Input: part model. Units: mm. Frame: model coordinates. A direction names the side the tool comes from. Give positions to 0.01 mm unless a question says otherwise; leave off trailing zeros. Loops run counter-clockwise (first coordinate to the right, second up) from the corner with the lowest first, then second, coordinate; pieces in that order, holes last. Notation, with made-up numbers: M 49.5,71 L 108.5,71 A21 ccw 108.5,104 Z; hole C -30.75,71.5 d2. An arc over 180 degrees is marked long. One line per item, written item: value. Start each with the question number.
(1) Access query for faces 4 (the flat face through (0, -27.5, 1)), 5 (the flat face through (32.5, 0, -12)), 6 (the flat face through (-47, 0, -20)), 7 (the cylindrical face through (-2.38, -10.74, 2.54)), 8 (the flat face through (37.5, 0, -7)). Directions: +Z, -Z, +X, -X, +Y, -Y. A direction counts if a zero-diameter tool reaches every point of the face in a straight line with its end or side. Return the directions, or none.
(2) Section B-B on z = -12.25. Output: boundary loops of the cut face in (x, y).
(3) Pull-direction query (X, two-part tool) for faces 1 (the flat face through (-1, -12, 5)), 2 (the flat face through (-37.5, 0, -8)), 3 (the flat face through (-32.5, 0, -12)); classes: released by +X, released by -X, zero draft, split by the parting line, or undercut.
(4) Section C-C on x = 25. Output: boundary loops of the cut face in (y, z).
(5) Section D-D on y = 8.5. Output: boundary loops of the cut face in (x, z), plus the area to 3 significant figures.
(6) Section A-A on x = -47.5. Output: boundary loops of the cut face in (y, z), plus the area to 3 significant figures.
(7) Pin query (flat end, axial travel): P1, Ø6, axis at x = -51, y = 10.5, coming from the +Z side; P2, Ø12.5, axis at y = -1.5, z = -5.5, coming from the -X side; P3, Ø4, axis at x = 25, y = 17.5, coming from the -Z side. Return the tip coordinate at first contact, or that it passes through.
(8) Ray query, line 1 along X through (y, z) = (15.5, -23.1); line 2 along Y through (x, z) = (0, 1.9); line 3 along Y through (x, z) = (47.5, -23.75). Return the intervals inside material, ascending. Write a range as from..to.
```python
from build123d import *

# Parameters (mm, degrees)
SKETCH1_W                                      = 75
SKETCH1_H                                      = 55
BOSS_EXTRUDE1_DEPTH                            = 5
SKETCH2_W                                      = 5
SKETCH2_H                                      = 55
BOSS_EXTRUDE2_DEPTH                            = 25
CUT_EXTRUDE1_REACH                             = 32
SKETCH3_R                                      = 5
SKETCH3_R_2                                    = 1.5
SKETCH3_R_3                                    = 11
SKETCH4_W                                      = 5
SKETCH4_H                                      = 55
BOSS_EXTRUDE3_DEPTH                            = 20
SKETCH5_W                                      = 5
SKETCH5_H                                      = 55
BOSS_EXTRUDE4_DEPTH                            = 20
M2_D_Z_BA_L_MAKINE_VIDAS_IN_HAV_A1_D           = 2.4
M2_D_Z_BA_L_MAKINE_VIDAS_IN_HAV_A1_CSINK_D     = 4.4
M2_D_Z_BA_L_MAKINE_VIDAS_IN_HAV_A1_CSINK_ANGLE = 90


with BuildPart() as part:
    # Sketch1 → Boss-Extrude1 (new body)
    with BuildSketch(Plane.XY):
        Rectangle(SKETCH1_W, SKETCH1_H)
    extrude(amount=BOSS_EXTRUDE1_DEPTH)

    # Sketch2 → Boss-Extrude2 (add)
    with BuildSketch(Plane(origin=(0, 0, 0), x_dir=(-1, 0, 0), z_dir=(0, 0, -1))):
        with Locations((-35, 0)):
            Rectangle(SKETCH2_W, SKETCH2_H)
        with Locations((35, 0)):
            Rectangle(SKETCH2_W, SKETCH2_H)
    extrude(amount=BOSS_EXTRUDE2_DEPTH)

    # Sketch3 → Cut-Extrude1 (cut, up to next)
    with BuildSketch(Plane.XY.offset(5), mode=Mode.PRIVATE) as cut_extrude1_sk1:
        with Locations((0, 17.5)):
            Circle(SKETCH3_R)
    cut_extrude1_tool1 = extrude(cut_extrude1_sk1.sketch, amount=-CUT_EXTRUDE1_REACH, mode=Mode.PRIVATE) & part.part
    add(cut_extrude1_tool1.solids().sort_by_distance((0, 17.5, 5))[0], mode=Mode.SUBTRACT)
    # Sketch3 → Cut-Extrude1 (cut, up to next)
    with BuildSketch(Plane.XY.offset(5), mode=Mode.PRIVATE) as cut_extrude1_sk2:
        with Locations((-25, 17.5)):
            Circle(SKETCH3_R_2)
    cut_extrude1_tool2 = extrude(cut_extrude1_sk2.sketch, amount=-CUT_EXTRUDE1_REACH, mode=Mode.PRIVATE) & part.part
    add(cut_extrude1_tool2.solids().sort_by_distance((-25, 17.5, 5))[0], mode=Mode.SUBTRACT)
    # Sketch3 → Cut-Extrude1 (cut, up to next)
    with BuildSketch(Plane.XY.offset(5), mode=Mode.PRIVATE) as cut_extrude1_sk3:
        with Locations((25, 17.5)):
            Circle(SKETCH3_R_2)
    cut_extrude1_tool3 = extrude(cut_extrude1_sk3.sketch, amount=-CUT_EXTRUDE1_REACH, mode=Mode.PRIVATE) & part.part
    add(cut_extrude1_tool3.solids().sort_by_distance((25, 17.5, 5))[0], mode=Mode.SUBTRACT)
    # Sketch3 → Cut-Extrude1 (cut, up to next)
    with BuildSketch(Plane.XY.offset(5), mode=Mode.PRIVATE) as cut_extrude1_sk4:
        Circle(SKETCH3_R_3)
    cut_extrude1_tool4 = extrude(cut_extrude1_sk4.sketch, amount=-CUT_EXTRUDE1_REACH, mode=Mode.PRIVATE) & part.part
    add(cut_extrude1_tool4.solids().sort_by_distance((0, 0, 5))[0], mode=Mode.SUBTRACT)

    # Sketch4 → Boss-Extrude3 (add)
    with BuildSketch(Plane(origin=(37.5, 0, 0), x_dir=(0, 0, -1), z_dir=(1, 0, 0))):
        with Locations((22.5, 0)):
            Rectangle(SKETCH4_W, SKETCH4_H)
    extrude(amount=BOSS_EXTRUDE3_DEPTH)

    # Sketch5 → Boss-Extrude4 (add)
    with BuildSketch(Plane.ZY.offset(37.5)):
        with Locations((-22.5, 0)):
            Rectangle(SKETCH5_W, SKETCH5_H)
    extrude(amount=BOSS_EXTRUDE4_DEPTH)

    # M2 Düz Başlı Makine Vidası İçin Havşa1 (through all)
    with Locations(Plane.XY.offset(-20)):
        with Locations((-47.5, 15.5), (-47.5, -15.5), (47.5, 15.5), (47.5, -15.5)):
            CounterSinkHole(M2_D_Z_BA_L_MAKINE_VIDAS_IN_HAV_A1_D / 2, M2_D_Z_BA_L_MAKINE_VIDAS_IN_HAV_A1_CSINK_D / 2, counter_sink_angle=M2_D_Z_BA_L_MAKINE_VIDAS_IN_HAV_A1_CSINK_ANGLE)


solid = part.part
```
Output values:
1. face 4: +Z, -Z, +X, -X, -Y
1. face 5: -Z, +Y, -Y
1. face 6: +Z, -X, +Y, -Y
1. face 7: +Z, -Z
1. face 8: +Z, +X, +Y, -Y
2. outline: M -37.5,-27.5 L -32.5,-27.5 L -32.5,27.5 L -37.5,27.5 Z; M 32.5,-27.5 L 37.5,-27.5 L 37.5,27.5 L 32.5,27.5 Z
3. face 1: zero draft
3. face 2: released by -X
3. face 3: undercut
4. outline: M -27.5,0 L 16,0 L 16,5 L -27.5,5 Z; M 19,0 L 27.5,0 L 27.5,5 L 19,5 Z
5. outline: M -57.5,-25 L -32.5,-25 L -32.5,0 L -6.98,0 L -6.98,5 L -37.5,5 L -37.5,-20 L -57.5,-20 Z; M 6.98,0 L 32.5,0 L 32.5,-25 L 57.5,-25 L 57.5,-20 L 37.5,-20 L 37.5,5 L 6.98,5 Z
5. area: 755 mm²
6. outline: M -27.5,-25 L -16.7,-25 L -16.7,-21 L -17.7,-20 L -27.5,-20 Z; M -14.3,-25 L 14.3,-25 L 14.3,-21 L 13.3,-20 L -13.3,-20 L -14.3,-21 Z; M 16.7,-25 L 27.5,-25 L 27.5,-20 L 17.7,-20 L 16.7,-21 Z
6. area: 249 mm²
7. P1: stops at z = -20
7. P2: stops at x = -37.5
7. P3: stops at z = 0
8. line 1: x = -57.5..-48.7, -46.3..-32.5, 32.5..46.3, 48.7..57.5
8. line 2: y = -27.5..-11, 11..12.5, 22.5..27.5
8. line 3: y = -27.5..-16.7, -14.3..14.3, 16.7..27.5
